```python
from build123d import *

# Parameters (mm, degrees)
SKETCH_1_R          = 2.5
EXTRUDE_1_DEPTH     = 60
CUT_EXTRUDE_START   = -15
CUT_EXTRUDE_1_DEPTH = 15
CHAMFER_1_SIZE      = 0.5


with BuildPart() as part:
    # Эскиз1 → Бобышка-Вытянуть1 (new body)
    with BuildSketch(Plane(origin=(0, 0, 0), x_dir=(1, 0, 0), z_dir=(0, 1, 0))):
        with Locations(Location((0, 0, 0), (0, 0, 270))):
            Circle(SKETCH_1_R)
    extrude(amount=EXTRUDE_1_DEPTH)

    # Эскиз2 → Вырез-Вытянуть1 (cut)
    with BuildSketch(Plane(origin=(0, 60, 0), x_dir=(1, 0, 0), z_dir=(0, 1, 0)).offset(CUT_EXTRUDE_START)):
        with BuildLine():
            Line((-1.5, 2), (1.5, 2))
            ThreePointArc((1.5, 2), (0, 2.5), (-1.5, 2))
        make_face()
    extrude(amount=CUT_EXTRUDE_1_DEPTH, mode=Mode.SUBTRACT)

    # Фаска1
    chamfer_1_edges = [part.edges().sort_by_distance(p)[0] for p in [
        (-2.371708245, 60, 0.790569415),
        (0, 0, -2.5),
    ]]
    chamfer(chamfer_1_edges, length=CHAMFER_1_SIZE - 0.0001)  # a hair under: the kernel refuses the full size


solid = part.part
```
Geometry check sheet. Reference: the model listing, model coordinates, mm. A direction names the side the tool comes from. Coordinates: 2 decimals unless noted, no trailing zeros. Write each loop counter-clockwise with the first axis right and the second up, starting at its lowest first coordinate (ties: lowest second). Pieces come first, ordered by that corner, then holes. Notation, with made-up numbers: (-40, -6.75) -> (-21, -6.75) arc R18 ccw to (-21, 4.25) -> close; hole circle Ø3 at (42, 87). An arc over 180 degrees is marked (long way). Use CSV: the item, a comma, the result in double quotes. Start each with the question number.
Item 1: Set-up check for faces 1 (the flat face through (0, 52, -2)), 2 (the cylindrical face through (0.751, 29.587, 2.385)): record each of +Z, -Z, +X, -X, +Y, -Y from which the full face is reachable in a straight line by a thin tool's end or side.
Item 2: Thickness scan on line 1 (X direction, y = 5, z = -0.2); line 2 (Z direction, x = -1.05, y = 28.5); line 3 (Y direction, x = 1.65, z = 1.2). Record the ranges inside material, lowest first.
Item 3: Cross-section at A-A, the plane y = 56. Record the cut outline in (x, z).
Item 4: Depth check by flat-ended pin: pin 1 Ø1 at (y, z) = (34, -2) entering from +X; pin 2 Ø0.5 at (x, z) = (-0.5, -2.5) entering from +Y; pin 3 Ø1 at (y, z) = (18, 1.5) entering from -X. Enter the tip coordinate at first touch or a pass-through.
Item 5: Cross-section at B-B, the plane y = 30. Record the cut outline in (x, z), plus the area to 3 significant figures.
Answers:
1,face 1,"-Z, +X, -X, +Y"
1,face 2,"+Y, -Y"
2,line 1,"-2.49 to 2.49"
2,line 2,"-2.27 to 2.27"
2,line 3,"0.04 to 59.96"
3,outline,"(-1.5, -2) -> (1.5, -2) arc R2.5 ccw (long way) to start"
4,pin 1,"x = 2"
4,pin 2,"y = 45"
4,pin 3,"x = -2.29"
5,outline,"circle Ø5 at (0, 0)"
5,area,"19.6 mm^2"
